Geometry check sheet. Reference: the model listing, model coordinates, mm. Face numbers are marked on the shaded views. A direction names the side the tool comes from. Give positions to 0.01 mm unless a question says otherwise; leave off trailing zeros. Order: outer loops, then holes, each group sorted by start corner. A loop starts at its lowest first (then second) coordinate and runs counter-clockwise, first axis right, second up.
```python
from build123d import *

# Parameters (mm, degrees)
SKETCH_1_W          = 18
SKETCH_1_H          = 18
EXTRUDE_1_DEPTH     = 5
SKETCH_2_R          = 8
CUT_EXTRUDE_1_DEPTH = 5
SKETCH_3_W          = 18
SKETCH_3_H          = 25
EXTRUDE_2_DEPTH     = 5
SKETCH_4_W          = 18
SKETCH_4_H          = 5
EXTRUDE_3_DEPTH     = 18
SKETCH_5_R          = 8
CUT_EXTRUDE_2_DEPTH = 18


with BuildPart() as part:
    # 草图1 → 凸台-拉伸1 (new body)
    with BuildSketch(Plane.XY):
        Rectangle(SKETCH_1_W, SKETCH_1_H)
    extrude(amount=EXTRUDE_1_DEPTH)

    # 草图2 → 切除-拉伸1 (cut)
    with BuildSketch(Plane.XY.offset(5)):
        Circle(SKETCH_2_R)
    extrude(amount=-CUT_EXTRUDE_1_DEPTH, mode=Mode.SUBTRACT)

    # 草图3 → 凸台-拉伸2 (add)
    with BuildSketch(Plane(origin=(0, 9, 0), x_dir=(1, 0, 0), z_dir=(0, 1, 0))):
        with Locations((0, 7.5)):
            Rectangle(SKETCH_3_W, SKETCH_3_H)
    extrude(amount=EXTRUDE_2_DEPTH)

    # 草图4 → 凸台-拉伸3 (add)
    with BuildSketch(Plane.XZ.offset(-9)):
        with Locations((0, -17.5)):
            Rectangle(SKETCH_4_W, SKETCH_4_H)
    extrude(amount=EXTRUDE_3_DEPTH)

    # 草图5 → 切除-拉伸2 (cut)
    with BuildSketch(Plane.XY.offset(-15)):
        Circle(SKETCH_5_R)
    extrude(amount=-CUT_EXTRUDE_2_DEPTH, mode=Mode.SUBTRACT)


solid = part.part
```
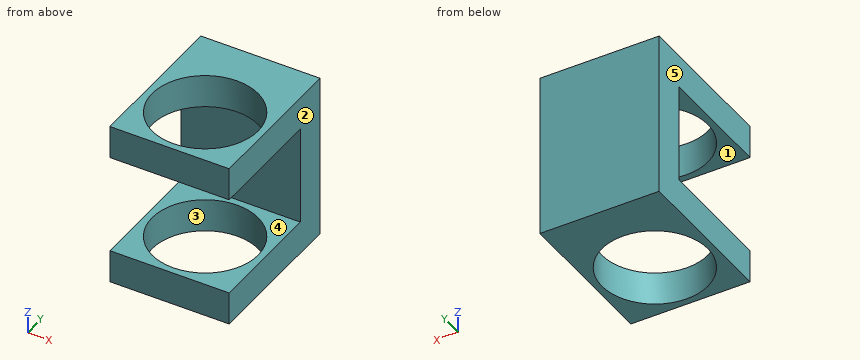
Q1. Release check for a two-part mould opening along X. For the marked faces 1, 2 and 3 record: pulls with the +X half, pulls with the -X half, needs draft (parallel to the pull), parting line crosses it, or undercut.
Q2. Cross-section at C-C, the plane z = 1.75. Record the boundary of the cut face in (x, y).
Q3. Cross-section at A-A, the plane y = 0. Record the boundary of the cut face in (x, z), and give its area (3 significant figures).
Q4. Thickness scan on L1, parallel to Y at x = 0, z = 3.2; L2, parallel to X at y = 0.25, z = -15.75; L3, parallel to Z at x = 7, y = 6.25. Record the ranges inside material, lowest first.
Q5. Access from +Z, -Z, +X, -X, +Y, -Y to the whole of each face (thin tool, end or side, straight path). Record for the marked faces 4 and 5.
Q6. Cross-section at D-D, the plane y = -5.5. Record the boundary of the cut face in (x, z), and give its area (3 significant figures).
Q7. Gauge pin test, flat end, axial feed: P1, Ø7.5, axis at x = -2.5, z = -10.5, coming from the -Y side. Record the tip position at first contact, or that the pin passes through.
Q8. Cross-section at B-B, the plane x = 0. Record the boundary of the cut face in (y, z).
Answers follow:
1. face 1: needs draft
1. face 2: pulls with the +X half
1. face 3: undercut
2. outline: (-9, -9) - (9, -9) - (9, 14) - (-9, 14) - close; hole circle Ø16 at (0, 0)
3. outline: (-9, -20) - (-8, -20) - (-8, -15) - (-9, -15) - close; (-9, 0) - (-8, 0) - (-8, 5) - (-9, 5) - close; (8, -20) - (9, -20) - (9, -15) - (8, -15) - close; (8, 0) - (9, 0) - (9, 5) - (8, 5) - close
3. area: 20.0 mm2
4. L1: y = -9 to -8, 8 to 14
4. L2: x = -9 to -8, 8 to 9
4. L3: z = -20 to -15, 0 to 5
5. face 4: +X, -X, -Y
5. face 5: +Z, -Z, -X, +Y, -Y
6. outline: (-9, -20) - (-5.81, -20) - (-5.81, -15) - (-9, -15) - close; (-9, 0) - (-5.81, 0) - (-5.81, 5) - (-9, 5) - close; (5.81, -20) - (9, -20) - (9, -15) - (5.81, -15) - close; (5.81, 0) - (9, 0) - (9, 5) - (5.81, 5) - close
6. area: 63.8 mm2
7. P1: stops at y = 9
8. outline: (-9, -20) - (-8, -20) - (-8, -15) - (-9, -15) - close; (-9, 0) - (-8, 0) - (-8, 5) - (-9, 5) - close; (8, -20) - (14, -20) - (14, 5) - (8, 5) - (8, 0) - (9, 0) - (9, -15) - (8, -15) - close
